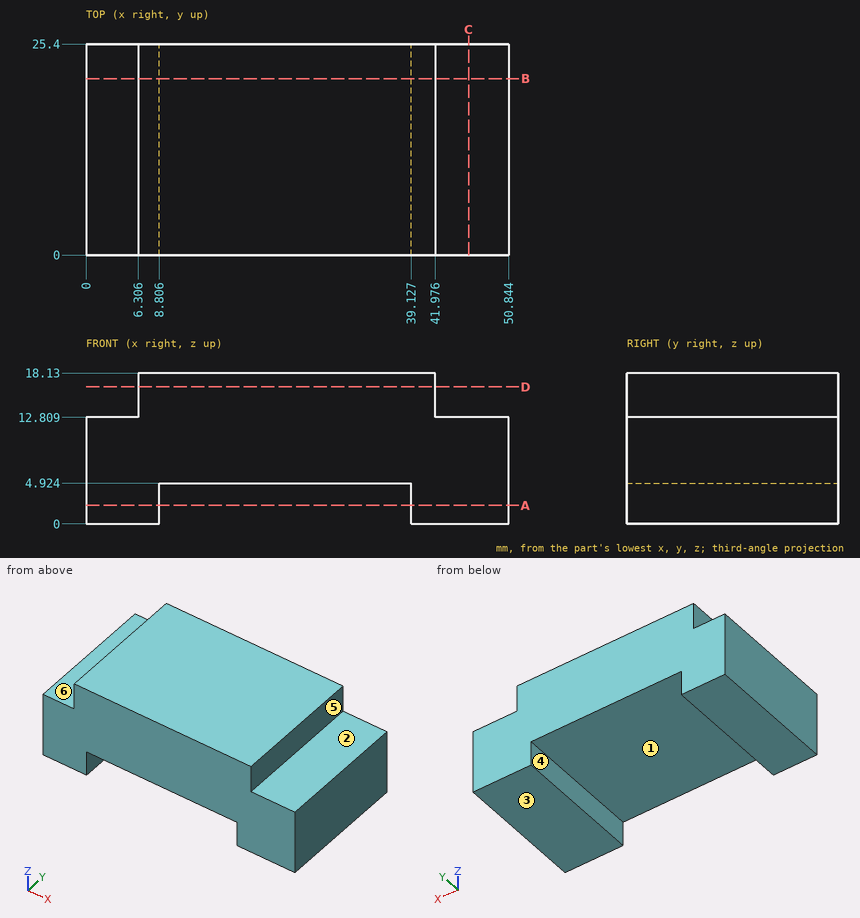
For this review, use the dimensioned drawing (mm, ordinates from the lowest corner) and the shaded views. A direction names the side the tool comes from. Give positions to 0.01 mm unless a question says otherwise; leave off trailing zeros. Order: outer loops, then holes, each group sorted by start corner. A loop starts at its lowest first (then second) coordinate and runs counter-clockwise, first axis right, second up. Notation, with made-up numbers: M 38,35 L 70,35 A27 ccw 70,67 Z; hole C 59.25,-6 d9. An arc over 180 degrees is marked long. Use one line per item in the form item = value. Start each with the question number.
Item 1: We need section D-D on z = 16.5. Give the boundary of the cut face in (x, y) (1 decimal).
Item 2: The part is to be moulded in two halves that separate along X. For the marked faces 4, 5 and 6, say which applies: pulls with the +X half, pulls with the -X half, needs draft (parallel to the pull), parting line crosses it, or undercut.
Item 3: For the marked faces 1, 2 and 3, list the 3-axis set-ups (+Z, -Z, +X, -X, +Y, -Y) from which the entire face can be reached by the end or side of a thin tool; tool diameter is ignored.
Item 4: We need section B-B on y = 21.25. Give the boundary of the cut face in (x, z) (1 decimal).
Item 5: To check wall thickness, follow line 1 along X through (y, z) = (6.25, 2.5) (1 decimal); line 2 along Z through (x, y) = (34.5, 23) (1 decimal); line 3 along Z through (x, y) = (44.5, 10.25). State the ranges of each line that lie inside material, in increasing order. Write a range as from..to.
Item 6: Insertion check: pin 1 Ø1.6 at (y, z) = (18, 16.5) entering from +X; pin 2 Ø4.5 at (x, y) = (47, 11) entering from +Z; pin 3 Ø2 at (x, y) = (12.5, 12) entering from -Z. Each pin has a flat end and moves straight along its axis. Give the tip position at first contact, or say it passes through.
Item 7: We need section A-A on z = 2.25. Give the boundary of the cut face in (x, y) (1 decimal), plus the area to 3 significant figures.
Item 8: We need section C-C on x = 46. Give the boundary of the cut face in (y, z).
Completed:
q1.outline = M 6.3,0 L 42,0 L 42,25.4 L 6.3,25.4 Z
q2.face_4 = undercut
q2.face_5 = pulls with the +X half
q2.face_6 = needs draft
q3.face_1 = -Z, +Y, -Y
q3.face_2 = +Z, +X, +Y, -Y
q3.face_3 = -Z, +X, -X, +Y, -Y
q4.outline = M 0,0 L 8.8,0 L 8.8,4.9 L 39.1,4.9 L 39.1,0 L 50.8,0 L 50.8,12.8 L 42,12.8 L 42,18.1 L 6.3,18.1 L 6.3,12.8 L 0,12.8 Z
q5.line_1 = 0..8.8, 39.1..50.8
q5.line_2 = 4.9..18.1
q5.line_3 = 0..12.81
q6.pin_1 = 41.98
q6.pin_2 = 12.81
q6.pin_3 = 4.92
q7.outline = M 0,0 L 8.8,0 L 8.8,25.4 L 0,25.4 Z; M 39.1,0 L 50.8,0 L 50.8,25.4 L 39.1,25.4 Z
q7.area = 521 mm²
q8.outline = M 0,0 L 25.4,0 L 25.4,12.81 L 0,12.81 Z
